```python
from build123d import *

# Parameters (mm, degrees)
F1_DEPTH = 1.25
F3_DEPTH = 3.6
F4_R     = 3
F5_DEPTH = 5
F5_TAPER = 3


with BuildPart() as f1:
    # F0 (on Front) → F1 (new body, symmetric)
    with BuildSketch(Plane.XZ):
        Polygon((3.5, 0.5295912741), (1, 0.9704087259), (-1, 0.9704087259), (-3.5, 0.5295912741), (-3.5, -0.9704087259), (0, -0.9704087259), (3.5, -0.9704087259), align=None)
    extrude(amount=F1_DEPTH, both=True)

    # F2 (on face) → F3 (join)
    with BuildSketch(Plane.XY.offset(0.9704087259)):
        with BuildLine():
            Line((1, -0.75), (1, 0.75))
            ThreePointArc((1, 0.75), (0.5590169944, 1.1180339887), (0, 1.25))
            ThreePointArc((0, 1.25), (-0.5590169944, 1.1180339887), (-1, 0.75))
            Line((-1, 0.75), (-1, -0.75))
            ThreePointArc((-1, -0.75), (-0.5590169944, -1.1180339887), (0, -1.25))
            ThreePointArc((0, -1.25), (0.5590169944, -1.1180339887), (1, -0.75))
        make_face()
    extrude(amount=F3_DEPTH)

    # F4 (on face) → F5 (join)
    with BuildSketch(Plane.XY.offset(4.5704087259)):
        Circle(F4_R)
        with BuildLine():
            Line((1, 0.75), (1, -0.75))
            ThreePointArc((1, -0.75), (0, -1.25), (-1, -0.75))
            Line((-1, -0.75), (-1, 0.75))
            ThreePointArc((-1, 0.75), (0, 1.25), (1, 0.75))
        make_face(mode=Mode.SUBTRACT)
        with BuildLine():
            ThreePointArc((-1, -0.75), (0, -1.25), (1, -0.75))
            Line((1, -0.75), (1, 0.75))
            ThreePointArc((1, 0.75), (0, 1.25), (-1, 0.75))
            Line((-1, 0.75), (-1, -0.75))
        make_face()
    extrude(amount=F5_DEPTH, taper=F5_TAPER)


solid = f1.part
```
The model under review builds one solid part; all positions refer to its coordinate system, in mm. A direction names the side the tool comes from. Give positions to 0.01 mm unless a question says otherwise; leave off trailing zeros. Write each loop counter-clockwise with the first axis right and the second up, starting at its lowest first coordinate (ties: lowest second). Pieces come first, ordered by that corner, then holes. Notation, with made-up numbers: M 44.5,67.5 L 77.5,67.5 A26 cw 77.5,101.5 Z; hole C 86,49.25 d6. An arc over 180 degrees is marked long. Write item = value, one per line. Start each with the question number.
Q1. We need section B-B (y = 0). State the section outline as (x, z) points, plus the area to 3 significant figures.
Q2. We need section D-D (z = 5.5). State the section outline as (x, y) points, plus the area to 3 significant figures.
Q3. For line 1 (Z direction, x = 1, y = 2.5); line 2 (Y direction, x = 3, z = 0.25); line 3 (Z direction, x = -2, y = -1), list the stretches that pass through material, from the lowest coordinate up.
Q4. We need section A-A (z = 2.25). State the section outline as (x, y) points.
Q5. We need section C-C (z = 7). State the section outline as (x, y) points, plus the area to 3 significant figures.
Q6. Clearance check with flat-ended pins moving along their axes: pin 1 (2 mm diameter, centred on y = 2.5, z = 7, fed in from -X); pin 2 (0.6 mm diameter, centred on x = -0.5, z = -0.5, fed in from -Y); pin 3 (0.8 mm diameter, centred on y = -0.5, z = 3, fed in from -X). State where each tip first meets the part, or that it passes through.
Q7. Machinability: for faces 1 (the face through (1.3, 0, 4.57)), 2 (the face through (-1, 0, 3)), 3 (the face through (0, -1.25, 0)), 4 (the face through (2.267, -0.018, 0.747)), which of the approach directions +Z, -Z, +X, -X, +Y, -Y give a long, thin tool a straight path to every point of the face, cutting with its end or side? Answer none if there is none.
Result set:
q1.outline = M -3.5,-0.97 L 3.5,-0.97 L 3.5,0.53 L 1,0.97 L 1,4.57 L 3,4.57 L 2.74,9.57 L -2.74,9.57 L -3,4.57 L -1,4.57 L -1,0.97 L -3.5,0.53 Z
q1.area = 48.4 mm2
q2.outline = C 0,0 d5.9
q2.area = 27.4 mm2
q3.line_1 = 4.57 to 9.57
q3.line_2 = -1.25 to 1.25
q3.line_3 = -0.97 to 0.79, 4.57 to 9.57
q4.outline = M -1,-0.75 A1.25 ccw 1,-0.75 L 1,0.75 A1.25 ccw -1,0.75 Z
q5.outline = C 0,0 d5.75
q5.area = 25.9 mm2
q6.pin_1 = -2.45
q6.pin_2 = -1.25
q6.pin_3 = -1
q7.face_1 = none
q7.face_2 = -X, +Y, -Y
q7.face_3 = -Z, +X, -X, -Y
q7.face_4 = +X, +Y, -Y
